Part model, mm, in its own coordinate system. A direction names the side the tool comes from. Round coordinates to 2 decimals unless told otherwise and drop trailing zeros. Loops run counter-clockwise (first coordinate to the right, second up) from the corner with the lowest first, then second, coordinate; pieces in that order, holes last. Notation, with made-up numbers: M 64,-38.5 L 97,-38.5 A20 ccw 97,-10.5 Z; hole C 26,52.5 d10. An arc over 180 degrees is marked long. Answer as CSV lines item,"result". Start each with the question number.
Item 1: Band-saw the part on C-C (x = -35). Give the cut face in (y, z).
Item 2: Which spindle directions (+Z, -Z, +X, -X, +Y, -Y) get a long thin tool onto all of the face, cutting with end or side? Do faces 4 (the cylindrical face through (25.566, -21.612, 4.597)), 5 (the flat face through (17.5, 6, 13)), 6 (the flat face through (37, 7, 13.85)), 7 (the flat face through (53, 7, -13.85)). Say none if no direction does.
Item 3: Band-saw the part on B-B (x = 14.5). Give the cut face in (y, z), and give its area (3 significant figures).
Item 4: Wall check: line 1 (X direction, y = -3.5, z = -0.5); line 2 (X direction, y = -1, z = 8); line 3 (X direction, y = 4.5, z = -8). Give the ranges that are in metal, low to high.
Item 5: Drop flat-ended pins along their axis: pin 1 Ø1.6 at (x, z) = (54.5, -15.5) entering from -Y; pin 2 Ø5.5 at (x, z) = (-2, 15) entering from +Y; pin 3 Ø5 at (x, y) = (-34, -16.5) entering from +Z. Give the stop position or say it passes through.
Item 6: Band-saw the part on D-D (y = -16.5). Give the cut face in (x, z) (3 decimals), and give its area (3 significant figures).
Item 7: Mould opens along X. For faces 1 (the flat face through (23.94, -24.71, 9.26)), 2 (the flat face through (-38, -3, -15)), 3 (the cylindrical face through (57, 5, 13)) say: pulls with the +X half, pulls with the -X half, needs draft (parallel to the pull), parting line crosses it, or undercut.
Item 8: Band-saw the part on A-A (z = -2). Give the cut face in (x, y), and give its area (3 significant figures).
```python
from build123d import *

# Parameters (mm, degrees)
BOSS_EXTRUDE1_DEPTH                             = 10
CSK_FOR_M4_FLAT_HEAD_MACHINE_SCREW1_D           = 4
CSK_FOR_M4_FLAT_HEAD_MACHINE_SCREW1_DEPTH       = 53.798278762
CSK_FOR_M4_FLAT_HEAD_MACHINE_SCREW1_CSINK_D     = 7.6
CSK_FOR_M4_FLAT_HEAD_MACHINE_SCREW1_CSINK_ANGLE = 90
CSK_FOR_M4_FLAT_HEAD_MACHINE_SCREW1_TIP         = 1.201721238
FILLET1_R                                       = 4
BOSS_EXTRUDE2_DEPTH                             = 28
SKETCH6_W                                       = 40
SKETCH6_H                                       = 1.5
SKETCH6_H_2                                     = 2
BOSS_EXTRUDE3_DEPTH                             = 7
SKETCH7_W                                       = 20
SKETCH7_H                                       = 10
BOSS_EXTRUDE4_DEPTH                             = 20
CHAMFER1_SIZE                                   = 3.6
BOSS_EXTRUDE5_START                             = 10
SKETCH9_W                                       = 4
SKETCH9_H                                       = 28
BOSS_EXTRUDE5_DEPTH                             = 76
CHAMFER2_SIZE                                   = 11.5
SKETCH10_W                                      = 56
SKETCH10_H                                      = 7
CUT_EXTRUDE1_DEPTH                              = 14.56
CHAMFER3_SIZE                                   = 1.5
CHAMFER3_SIZE2                                  = 6.497213811
CSK_FOR_M4_FLAT_HEAD_MACHINE_SCREW2_D           = 4
CSK_FOR_M4_FLAT_HEAD_MACHINE_SCREW2_DEPTH       = 38.798278762
CSK_FOR_M4_FLAT_HEAD_MACHINE_SCREW2_CSINK_D     = 7.9
CSK_FOR_M4_FLAT_HEAD_MACHINE_SCREW2_CSINK_ANGLE = 90
CSK_FOR_M4_FLAT_HEAD_MACHINE_SCREW2_TIP         = 1.201721238
CUT_EXTRUDE2_DEPTH                              = 3.15
F_1_0MM_DOWEL_HOLE1_D                           = 3
F_1_0MM_DOWEL_HOLE1_DEPTH                       = 12.598709071
F_1_0MM_DOWEL_HOLE1_TIP                         = 0.901290929
CHAMFER4_SIZE                                   = 10
CUT_EXTRUDE3_DEPTH                              = 3.15
SKETCH17_W                                      = 5.7
SKETCH17_H                                      = 8
CUT_EXTRUDE4_DEPTH                              = 42
CUT_EXTRUDE5_DEPTH                              = 75.431176264
CUT_EXTRUDE5_DEPTH_BACK                         = 75.431176264
SKETCH18_W                                      = 35
SKETCH18_H                                      = 14
CUT_EXTRUDE6_DEPTH                              = 15
CSK_FOR_M4_SFHCS2_D                             = 4
CSK_FOR_M4_SFHCS2_DEPTH                         = 11
CSK_FOR_M4_SFHCS2_CSINK_D                       = 7.6
CSK_FOR_M4_SFHCS2_CSINK_ANGLE                   = 90
CSK_FOR_M4_SFHCS2_TIP                           = 1.201721238
CSK_FOR_M4_SFHCS3_D                             = 4
CSK_FOR_M4_SFHCS3_DEPTH                         = 16
CSK_FOR_M4_SFHCS3_CSINK_D                       = 7.9
CSK_FOR_M4_SFHCS3_CSINK_ANGLE                   = 90
CSK_FOR_M4_SFHCS3_TIP                           = 1.201721238
CUT_EXTRUDE7_DEPTH                              = 0.4


with BuildPart() as part:
    # Sketch1 → Boss-Extrude1 (new body)
    with BuildSketch(Plane(origin=(0, 0, 0), x_dir=(1, 0, 0), z_dir=(0, 1, 0))):
        Polygon((60, 17), (-60, 17), (-60, 10), (-28, 10), (-28, 0), (-20, 0), (-20, 10), (20, 10), (20, 0), (28, 0), (28, 10), (60, 10), align=None)
        Polygon((-20, 0), (-28, 0), (-28, -10), (-60, -10), (-60, -17), (60, -17), (60, -10), (28, -10), (28, 0), (20, 0), (20, -10), (-20, -10), align=None)
    extrude(amount=BOSS_EXTRUDE1_DEPTH)

    # CSK for M4 Flat Head Machine Screw1
    with Locations(Plane.XY.offset(17)):
        with Locations((-55, 5), (55, 5)):
            CounterSinkHole(CSK_FOR_M4_FLAT_HEAD_MACHINE_SCREW1_D / 2, CSK_FOR_M4_FLAT_HEAD_MACHINE_SCREW1_CSINK_D / 2, depth=CSK_FOR_M4_FLAT_HEAD_MACHINE_SCREW1_DEPTH, counter_sink_angle=CSK_FOR_M4_FLAT_HEAD_MACHINE_SCREW1_CSINK_ANGLE)
            with Locations((0, 0, -(CSK_FOR_M4_FLAT_HEAD_MACHINE_SCREW1_DEPTH + CSK_FOR_M4_FLAT_HEAD_MACHINE_SCREW1_TIP / 2))):  # 118° drill point
                Cone(0, CSK_FOR_M4_FLAT_HEAD_MACHINE_SCREW1_D / 2, CSK_FOR_M4_FLAT_HEAD_MACHINE_SCREW1_TIP, mode=Mode.SUBTRACT)

    # Fillet1
    fillet1_edges = [part.edges().sort_by_distance(p)[0] for p in [
        (60, 0, 13.5),
        (-60, 0, 13.5),
        (-60, 0, -13.5),
        (60, 0, -13.5),
        (60, 10, -13.5),
        (-60, 10, -13.5),
        (-60, 10, 13.5),
        (60, 10, 13.5),
    ]]
    fillet(fillet1_edges, radius=FILLET1_R)

    # Sketch5 → Boss-Extrude2 (add)
    with BuildSketch(Plane.XZ):
        Polygon((-28, 10), (-28, -17), (28, -17), (28, 10), (20, 10), (20, -10), (-20, -10), (-20, 10), align=None)
    extrude(amount=BOSS_EXTRUDE2_DEPTH)

    # Sketch6 → Boss-Extrude3 (add)
    with BuildSketch(Plane.XY.offset(10)):
        Polygon((-28, 0), (-28, -28), (28, -28), (28, 0), (20, 0), (20, -2.94), (-20, -2.94), (-20, 0), align=None)
        with Locations((0, -6.19)):
            Rectangle(SKETCH6_W, SKETCH6_H, mode=Mode.SUBTRACT)
        with Locations((0, -10.19)):
            Rectangle(SKETCH6_W, SKETCH6_H, mode=Mode.SUBTRACT)
        with Locations((0, -14.19)):
            Rectangle(SKETCH6_W, SKETCH6_H, mode=Mode.SUBTRACT)
        with Locations((0, -18.19)):
            Rectangle(SKETCH6_W, SKETCH6_H, mode=Mode.SUBTRACT)
        with Locations((0, -22.44)):
            Rectangle(SKETCH6_W, SKETCH6_H_2, mode=Mode.SUBTRACT)
    extrude(amount=BOSS_EXTRUDE3_DEPTH)

    # Sketch7 → Boss-Extrude4 (add)
    with BuildSketch(Plane.XY.offset(-10)):
        with Locations((38, 5)):
            Rectangle(SKETCH7_W, SKETCH7_H)
        with Locations((-38, 5)):
            Rectangle(SKETCH7_W, SKETCH7_H)
    extrude(amount=BOSS_EXTRUDE4_DEPTH)

    # Chamfer1
    chamfer1_edges = [part.edges().sort_by_distance(p)[0] for p in [
        (48, 10, 0),
        (48, 0, 0),
        (-48, 0, 0),
        (-48, 10, 0),
    ]]
    chamfer(chamfer1_edges, length=CHAMFER1_SIZE)

    # Sketch9 → Boss-Extrude5 (add)
    with BuildSketch(Plane.ZY.offset(28).offset(BOSS_EXTRUDE5_START)):
        with Locations((-15, -14)):
            Rectangle(SKETCH9_W, SKETCH9_H)
    extrude(amount=-BOSS_EXTRUDE5_DEPTH)

    # Chamfer2
    chamfer2_edges = [part.edges().sort_by_distance(p)[0] for p in [
        (38, -28, -15),
        (-38, -28, -15),
    ]]
    chamfer(chamfer2_edges, length=CHAMFER2_SIZE)

    # Sketch10 → Cut-Extrude1 (cut)
    with BuildSketch(Plane.XZ.offset(28)):
        with Locations((0, 13.5)):
            Rectangle(SKETCH10_W, SKETCH10_H)
    extrude(amount=-CUT_EXTRUDE1_DEPTH, mode=Mode.SUBTRACT)

    # Chamfer3
    chamfer3_edges = [part.edges().sort_by_distance(p)[0] for p in [
        (23.25, -28, 10),
        (-23.25, -28, 10),
    ]]
    chamfer3_side = [part.faces().sort_by_distance(p)[0] for p in [
        (0, -28, -16.405189106),
    ]]
    chamfer(chamfer3_edges, length=CHAMFER3_SIZE, length2=CHAMFER3_SIZE2, reference=chamfer3_side[0])

    # CSK for M4 Flat Head Machine Screw2
    with Locations(Plane(origin=(-695.683007616, 1385.247292614, -21), x_dir=(-1, 0, 0), z_dir=(0, 0, -1))):
        with Locations((-730.683007616, -1380.247292614), (-660.683007616, -1380.247292614)):
            CounterSinkHole(CSK_FOR_M4_FLAT_HEAD_MACHINE_SCREW2_D / 2, CSK_FOR_M4_FLAT_HEAD_MACHINE_SCREW2_CSINK_D / 2, depth=CSK_FOR_M4_FLAT_HEAD_MACHINE_SCREW2_DEPTH, counter_sink_angle=CSK_FOR_M4_FLAT_HEAD_MACHINE_SCREW2_CSINK_ANGLE)
            with Locations((0, 0, -(CSK_FOR_M4_FLAT_HEAD_MACHINE_SCREW2_DEPTH + CSK_FOR_M4_FLAT_HEAD_MACHINE_SCREW2_TIP / 2))):  # 118° drill point
                Cone(0, CSK_FOR_M4_FLAT_HEAD_MACHINE_SCREW2_D / 2, CSK_FOR_M4_FLAT_HEAD_MACHINE_SCREW2_TIP, mode=Mode.SUBTRACT)

    # Sketch13 → Cut-Extrude2 (cut)
    with BuildSketch(Plane.XY.offset(17)):
        Polygon((-31.016283143, 5), (-33.008141571, 8.45), (-36.991858429, 8.45), (-38.983716857, 5), (-36.991858429, 1.55), (-33.008141571, 1.55), align=None)
        Polygon((38.983716857, 5), (36.991858429, 8.45), (33.008141571, 8.45), (31.016283143, 5), (33.008141571, 1.55), (36.991858429, 1.55), align=None)
    extrude(amount=-CUT_EXTRUDE2_DEPTH, mode=Mode.SUBTRACT)

    # Ø1.0mm Dowel Hole1
    with Locations(Plane(origin=(0, -28, 0), x_dir=(-1, 0, 0), z_dir=(0, -1, 0))):
        with Locations((-24.134952034, 4.858), (-24.134952034, -5.048), (24.015, -5.048), (24.015, 4.858)):
            Hole(F_1_0MM_DOWEL_HOLE1_D / 2, depth=F_1_0MM_DOWEL_HOLE1_DEPTH)
            with Locations((0, 0, -(F_1_0MM_DOWEL_HOLE1_DEPTH + F_1_0MM_DOWEL_HOLE1_TIP / 2))):  # 118° drill point
                Cone(0, F_1_0MM_DOWEL_HOLE1_D / 2, F_1_0MM_DOWEL_HOLE1_TIP, mode=Mode.SUBTRACT)

    # Chamfer4
    chamfer4_edges = [part.edges().sort_by_distance(p)[0] for p in [
        (38, -16.5, -15),
        (-38, -16.5, -15),
    ]]
    chamfer(chamfer4_edges, length=CHAMFER4_SIZE)

    # Sketch16 → Cut-Extrude3 (cut)
    with BuildSketch(Plane(origin=(0, 0, -17), x_dir=(-1, 0, 0), z_dir=(0, 0, -1))):
        Polygon((51.016283143, 5), (53.008141571, 1.55), (56.991858429, 1.55), (58.983716857, 5), (56.991858429, 8.45), (53.008141571, 8.45), align=None)
        Polygon((-51.016283143, 5), (-53.008141571, 8.45), (-56.991858429, 8.45), (-58.983716857, 5), (-56.991858429, 1.55), (-53.008141571, 1.55), align=None)
    extrude(amount=-CUT_EXTRUDE3_DEPTH, mode=Mode.SUBTRACT)

    # Sketch17 → Cut-Extrude4 (cut)
    with BuildSketch(Plane.XZ.offset(28)):
        with Locations((20, -0.75)):
            Rectangle(SKETCH17_W, SKETCH17_H)
    extrude(amount=-CUT_EXTRUDE4_DEPTH, mode=Mode.SUBTRACT)

    # Sketch18 → Cut-Extrude5 (cut, two sides: drawn at the far end of the back side and taken through both)
    with BuildSketch(Plane.XY.offset(17).offset(-CUT_EXTRUDE5_DEPTH_BACK)):
        with Locations((0, 10)):
            Rectangle(SKETCH18_W, SKETCH18_H)
    extrude(amount=CUT_EXTRUDE5_DEPTH + CUT_EXTRUDE5_DEPTH_BACK, mode=Mode.SUBTRACT)

    # Sketch19 → Cut-Extrude6 (cut)
    with BuildSketch(Plane(origin=(-695.683007616, 1385.247292614, 25), x_dir=(1, 0, 0), z_dir=(0, 0, 1))):
        Polygon((667.683007616, -1396.089662241), (667.683007616, -1398.687292614), (671.683007616, -1398.687292614), align=None)
        Polygon((719.683007616, -1398.687292614), (723.683007616, -1398.687292614), (723.683007616, -1396.089662241), align=None)
    extrude(amount=-CUT_EXTRUDE6_DEPTH, mode=Mode.SUBTRACT)

    # CSK for M4 SFHCS2
    with Locations(Plane(origin=(-695.683007616, 1385.247292614, -10), x_dir=(1, 0, 0), z_dir=(0, 0, 1))):
        with Locations((681.183007616, -1407.747292614), (710.183007616, -1407.747292614)):
            CounterSinkHole(CSK_FOR_M4_SFHCS2_D / 2, CSK_FOR_M4_SFHCS2_CSINK_D / 2, depth=CSK_FOR_M4_SFHCS2_DEPTH, counter_sink_angle=CSK_FOR_M4_SFHCS2_CSINK_ANGLE)
            with Locations((0, 0, -(CSK_FOR_M4_SFHCS2_DEPTH + CSK_FOR_M4_SFHCS2_TIP / 2))):  # 118° drill point
                Cone(0, CSK_FOR_M4_SFHCS2_D / 2, CSK_FOR_M4_SFHCS2_TIP, mode=Mode.SUBTRACT)

    # CSK for M4 SFHCS3
    with Locations(Plane(origin=(-695.683007616, 1385.247292614, 25), x_dir=(1, 0, 0), z_dir=(0, 0, 1))):
        with Locations((672.933007616, -1385.668477427), (718.433007616, -1385.668477427)):
            CounterSinkHole(CSK_FOR_M4_SFHCS3_D / 2, CSK_FOR_M4_SFHCS3_CSINK_D / 2, depth=CSK_FOR_M4_SFHCS3_DEPTH, counter_sink_angle=CSK_FOR_M4_SFHCS3_CSINK_ANGLE)
            with Locations((0, 0, -(CSK_FOR_M4_SFHCS3_DEPTH + CSK_FOR_M4_SFHCS3_TIP / 2))):  # 118° drill point
                Cone(0, CSK_FOR_M4_SFHCS3_D / 2, CSK_FOR_M4_SFHCS3_TIP, mode=Mode.SUBTRACT)

    # Sketch26 → Cut-Extrude7 (cut)
    with BuildSketch(Plane.XY.offset(-10)):
        with BuildLine():
            Line((-48, 3.6), (-48, 6.4))
            Line((-48, 6.4), (-44.4, 10))
            Line((-44.4, 10), (-56, 10))
            ThreePointArc((-56, 10), (-58.828427125, 8.828427125), (-60, 6))
            Line((-60, 6), (-60, 4))
            ThreePointArc((-60, 4), (-58.828427125, 1.171572875), (-56, 0))
            Line((-56, 0), (-44.4, 0))
            Line((-44.4, 0), (-48, 3.6))
        make_face()
        with BuildLine():
            Line((48, 6.4), (48, 3.6))
            Line((48, 3.6), (44.4, 0))
            Line((44.4, 0), (56, 0))
            ThreePointArc((56, 0), (58.828427125, 1.171572875), (60, 4))
            Line((60, 4), (60, 6))
            ThreePointArc((60, 6), (58.828427125, 8.828427125), (56, 10))
            Line((56, 10), (44.4, 10))
            Line((44.4, 10), (48, 6.4))
        make_face()
    extrude(amount=-CUT_EXTRUDE7_DEPTH, mode=Mode.SUBTRACT)


solid = part.part
```
Answer block:
1,outline,"M -13.74,-17 L 3,-17 L 3,13.85 L 1.55,13.85 L 1.55,17 L 0,17 L 0,-13 L -13.74,-13 Z; M 7,-17 L 10,-17 L 10,17 L 8.45,17 L 8.45,13.85 L 7,13.85 Z"
2,face 4,"-Y"
2,face 5,"+Z, -Z, +Y"
2,face 6,"+Z"
2,face 7,"-Z"
3,outline,"M -28,-17 L -24.5,-17 L -24.5,-11.8 L -26.3,-10 L -28,-10 Z; M -20.5,-17 L 3,-17 L 3,-10 L -18.7,-10 L -20.5,-11.8 Z; M -13.44,10 L -10.94,10 L -10.94,17 L -13.44,17 Z; M -9.44,10 L -6.94,10 L -6.94,17 L -9.44,17 Z; M -5.44,10 L -2.94,10 L -2.94,17 L -5.44,17 Z; M 0,10 L 3,10 L 3,17 L 0,17 Z"
3,area,"259 mm^2"
4,line 1,"x = -28 to -20, 22.85 to 28"
4,line 2,"x = -28 to -20, 20 to 28"
4,line 3,"x = -48 to -36.94, -33.06 to -20, 20 to 33.06, 36.94 to 48"
5,pin 1,"stops at y = 0"
5,pin 2,"stops at y = 3"
5,pin 3,"stops at z = -13"
6,outline,"M -33.858,-17 L 33.858,-17 L 33.858,-13 L 28,-13 L 28,10 L 20,10 L 20,3.25 L 22.85,3.25 L 22.85,-4.084 A1.5 cw long 22.639,-4.75 L 20,-4.75 L 20,-10 L -20,-10 L -20,10 L -28,10 L -28,-13 L -33.858,-13 Z; hole C -24.015,-4.858 d3; hole C -24.015,5.048 d3; hole C 24.135,5.048 d3"
6,area,"708 mm^2"
7,face 1,"needs draft"
7,face 2,"pulls with the -X half"
7,face 3,"undercut"
8,outline,"M -48,3.6 L -44.4,0 L -28,0 L -28,-26.5 L -26.5,-28 L -20,-28 L -20,10 L -44.4,10 L -48,6.4 Z; M 22.85,-28 L 26.5,-28 L 28,-26.5 L 28,0 L 44.4,0 L 48,3.6 L 48,6.4 L 44.4,10 L 22.85,10 Z; hole C -35,5 d4; hole C 35,5 d4"
8,area,"846 mm^2"
